The listing builds one solid part. Answer for the finished solid, in the listing's coordinates (mm). A direction names the side the tool comes from. Coordinates: 2 decimals unless noted, no trailing zeros. Order: outer loops, then holes, each group sorted by start corner. A loop starts at its lowest first (then second) coordinate and runs counter-clockwise, first axis right, second up. Notation, with made-up numbers: M -33.75,79.25 L -7.75,79.25 A21 cw -7.75,93.25 Z; hole C 70.25,-13 d9. An arc over 180 degrees is marked long. One line per item, written item: value. Start each with the question number.
Q1. Each of these flat-tipped pins is pushed along its axis until it touches: pin 1 Ø10 at (x, z) = (10.5, -88.5) entering from +Y; pin 2 Ø2.5 at (x, y) = (20.5, 35) entering from -Z; pin 3 Ø4 at (y, z) = (4.5, -76.5) entering from -X. Where does it stop, or does it pass through?
Q2. For faces 1 (the flat face through (19, 12.7, -59)), 2 (the flat face through (8, 4, -7.62)), 3 (the flat face through (16, 69, -20.574)), 4 (the flat face through (15.24, 20, -46)), determine the directions among +Z, -Z, +X, -X, +Y, -Y from which every point of the face is accessible in a straight line to the end or side of a thin tool.
Q3. The part is cut by section A-A on z = -17. Give the vertices of the cut face in (x, y), then the cut area to 3 significant figures.
Q4. The part is cut by section D-D on x = 21.5. Give the vertices of the cut face in (y, z).
Q5. The part is cut by section B-B on y = 88. Give the vertices of the cut face in (x, z).
Q6. Straight lines are drawn through the part: line 1 along Y through (x, z) = (4.75, -6); line 2 along Y through (x, z) = (16, -21); line 3 along Z through (x, y) = (17.5, 72). For each, find the intervals that lie inside material, in ascending order. Write a range as [from, to].
Q7. The part is cut by section C-C on x = 8.75. Give the vertices of the cut face in (y, z), then the cut area to 3 significant figures.
Q8. Determine the mould class of faces 5 (the flat face through (9, 10, -106.68)), 6 (the flat face through (11, 10, -114.3)), 7 (the flat face through (8, 7.62, -4)) for opening direction Z: pulls with the +Z half, pulls with the -Z half, needs draft (parallel to the pull), parting line crosses it, or undercut.
```python
from build123d import *

# Parameters (mm, degrees)
F1_DEPTH = 22.86
F2_W     = 15.24
F2_H     = 119.38
F3_DEPTH = 106.68
F4_W     = 7.62
F4_H     = 7.62
F5_DEPTH = 15.24


with BuildPart() as f1:
    # F0 (on Right) → F1 (new body)
    with BuildSketch(Plane.YZ):
        Polygon((0, 0), (0, -114.3), (20.32, -114.3), (20.32, -20.574), (101.6, -20.574), (101.6, 0), (20.32, 0), align=None)
        Polygon((12.7, -106.68), (7.62, -106.68), (7.62, -7.62), (93.98, -7.62), (93.98, -12.954), (12.7, -12.954), align=None, mode=Mode.SUBTRACT)
    extrude(amount=F1_DEPTH)

    # F2 (on face) → F3 (cut)
    with BuildSketch(Plane.XY):
        with Locations((7.62, 34.29)):
            Rectangle(F2_W, F2_H)
    extrude(amount=-F3_DEPTH, mode=Mode.SUBTRACT)

    # F4 (on face) → F5 (join, through all)
    with BuildSketch(Plane(origin=(15.24, 0, 0), x_dir=(0, -1, 0), z_dir=(-1, 0, 0))):
        with Locations((-3.81, -3.81)):
            Rectangle(F4_W, F4_H)
    extrude(amount=F5_DEPTH)


solid = f1.part
```
Output:
1. pin 1: stops at y = 20.32
1. pin 2: stops at z = -20.57
1. pin 3: stops at x = 15.24
2. face 1: +X, -X
2. face 2: -X, -Y
2. face 3: -Z, +X, -X, +Y
2. face 4: +Z, -X, -Y
3. outline: M 0,93.98 L 15.24,93.98 L 15.24,12.7 L 22.86,12.7 L 22.86,101.6 L 0,101.6 Z; M 15.24,0 L 22.86,0 L 22.86,7.62 L 15.24,7.62 Z
3. area: 852 mm^2
4. outline: M 0,-114.3 L 20.32,-114.3 L 20.32,-20.57 L 101.6,-20.57 L 101.6,0 L 0,0 Z; hole M 7.62,-106.68 L 12.7,-106.68 L 12.7,-12.95 L 93.98,-12.95 L 93.98,-7.62 L 7.62,-7.62 Z
5. outline: M 15.24,-20.57 L 22.86,-20.57 L 22.86,-12.95 L 15.24,-12.95 Z; M 15.24,-7.62 L 22.86,-7.62 L 22.86,0 L 15.24,0 Z
6. line 1: y = [0, 7.62], [93.98, 101.6]
6. line 2: y = [0, 7.62], [12.7, 20.32]
6. line 3: z = [-20.57, -12.95], [-7.62, 0]
7. outline: M 0,-114.3 L 20.32,-114.3 L 20.32,-106.68 L 0,-106.68 Z; M 0,-7.62 L 7.62,-7.62 L 7.62,0 L 0,0 Z; M 93.98,-20.57 L 101.6,-20.57 L 101.6,0 L 93.98,0 Z
7. area: 370 mm^2
8. face 5: undercut
8. face 6: pulls with the -Z half
8. face 7: needs draft
